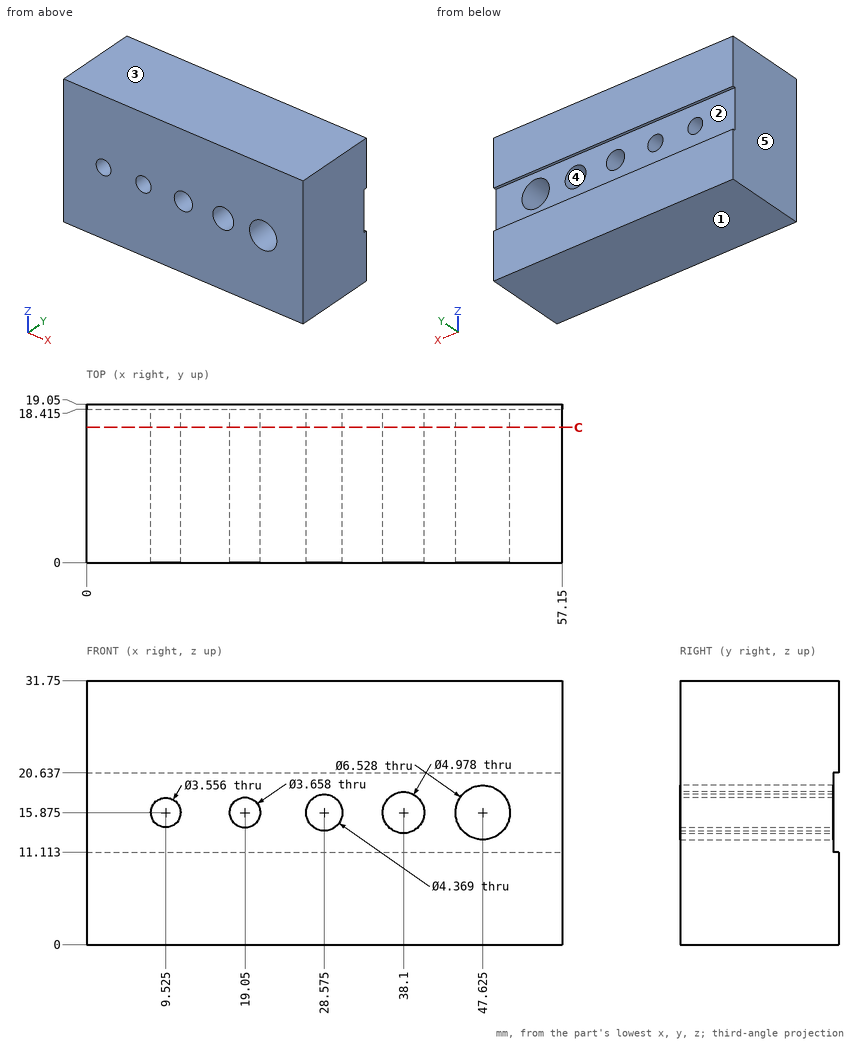
Job drawing, mm, ordinate dimensions from the low corner. One solid piece. A direction names the side the tool comes from. Round coordinates to 2 decimals unless told otherwise and drop trailing zeros.
Item 1: 3-axis set-ups, long thin cutter, end or side, ignore diameter. For the marked faces 1 and 2: which of +Z, -Z, +X, -X, +Y, -Y reach the whole face in a straight line?
Item 2: Cut at C-C, the plane y = 16.25. State how many separate pieces and enclosed holes the cut face has, then the cut area to 3 significant figures.
Item 3: Drop flat-ended pins along their axis: P1, Ø8, axis at x = 8.5, z = 26, coming from the -Y side; P2, Ø7, axis at x = 28.575, z = 15.875, coming from the +Y side (1 decimal); P3, Ø2, axis at x = 9.525, z = 15.875, coming from the +Y side. Give the stop position or say it passes through.
Item 4: Mould opens along Z. For the marked faces 3, 4 and 5 say: +Z half, -Z half, draft (parallel to the pull), parting line (faces both ways), or undercut.
Item 5: Drill centre lines: line 1 (Z direction, x = 38, y = 17.75); line 2 (Z direction, x = 19, y = 6); line 3 (Y direction, x = 46, z = 13) (1 decimal). Where is each one in solid material? Low to high.
A:
1. face 1: -Z, +X, -X, +Y, -Y
1. face 2: +X, -X, +Y
2. separate pieces: 1
2. enclosed holes: 5
2. area: 1,730 mm2
3. P1: stops at y = 0
3. P2: stops at y = 18.4
3. P3: passes through
4. face 3: +Z half
4. face 4: undercut
4. face 5: draft
5. line 1: z = 0 to 13.39, 18.36 to 31.75
5. line 2: z = 0 to 14.05, 17.7 to 31.75
5. line 3: y = 0 to 18.4
